Autodesk Inventor part; units mm, degrees
ref_plane "YZ Plane" through (0, 0, 0) normal (1, 0, 0) x (0, 1, 0)
ref_plane "XZ Plane" through (0, 0, 0) normal (0, 1, 0) x (-1, 0, 0)
ref_plane "XY Plane" through (0, 0, 0) normal (0, 0, 1) x (1, 0, 0)
sketch "Sketch1" plane through (0, 0, 0) normal (1, 0, 0) x (0, 1, 0)
  line L0 (-55.5791, 90.9825) -> (55.5791, 90.9825)
  line L1 (55.5791, 90.9825) -> (55.5791, -90.9825)
  line L2 (55.5791, -90.9825) -> (-55.5791, -90.9825)
  line L3 (-55.5791, -90.9825) -> (-55.5791, 90.9825)
  line L4 (-55.5791, 90.9825) -> (55.5791, -90.9825) construction
  line L5 (55.5791, 90.9825) -> (-55.5791, -90.9825) construction
  circle A0 centre (35.8863, -80.1209) radius 6.35
  arc A1 (28.845, 21.2348) -> (-35.1241, -7.4567) centre (35.8863, -80.1209) ccw construction
  arc A2 (28.1849, 30.7369) -> (-41.7813, -0.6445) centre (35.8863, -80.1209) ccw
  arc A3 (29.5052, 11.7327) -> (-28.4669, -14.269) centre (35.8863, -80.1209) ccw
  arc A4 (29.5052, 11.7327) -> (28.1849, 30.7369) centre (28.845, 21.2348) ccw
  arc A5 (-41.7813, -0.6445) -> (-28.4669, -14.269) centre (-35.1241, -7.4567) ccw
  circle A6 centre (28.845, 71.7808) radius 14.2875
  point P0 (0, 0)
  dimension "d2" = 12.7
  dimension "d3" = 101.6
  dimension "d4" = 19.05
  dimension "d5" = 28.575
  dimension "d9" = 50.546
  dimension "d10" = 0
  dimension "d11" = 181.965
  dimension "d12" = 111.1583
extrude "Extrusion1" add sketch "Sketch1" along normal blind 7.9375
properties part number "side_plate" material "Steel"
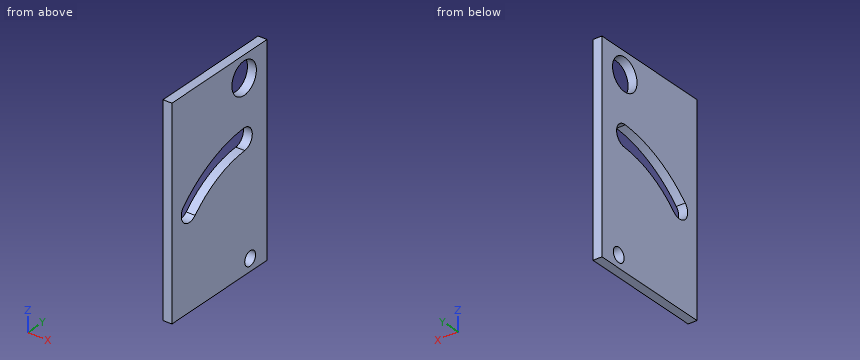
Can you work these out from the model? Positions are in its coordinate system, mm. Round coordinates to 2 decimals unless told otherwise and drop trailing zeros. Write each loop counter-clockwise with the first axis right and the second up, starting at its lowest first coordinate (ties: lowest second). Pieces come first, ordered by that corner, then holes. Notation, with made-up numbers: (-28.5, 24.25) - (-9.5, 24.25) arc R20 ccw to (-9.5, 61.25) - close; hole circle Ø8 at (17, -13). An arc over 180 degrees is marked (long way). Write each question's results on one line, items separated by ' | '. Start each with the question number.
1) Suppose I cut it at D-D (y = 23). List the corners of the cut face in (x, z) for me.
2) Suppose I cut it at B-B (z = -3). List the corners of the cut face in (x, y) for me, and give its area (3 significant figures).
3) Please list where these lines run through material, in increasing order: line 1 (Z direction, x = 2.5, y = 23.5); line 2 (Z direction, x = 2.5, y = 37.5); line 3 (Z direction, x = 7.5, y = 17).
4) Suppose I cut it at A-A (x = 3.25). Give the number of separate pieces and of enclosed holes in the cut face, and give its area (3 significant figures).
5) Suppose I cut it at C-C (y = 36). List the corners of the cut face in (x, z) for me, and give its area (3 significant figures).
Here are the results:
1) outline: (0, -90.98) - (7.94, -90.98) - (7.94, 11.05) - (0, 11.05) - close; (0, 30.25) - (7.94, 30.25) - (7.94, 58.74) - (0, 58.74) - close; (0, 84.82) - (7.94, 84.82) - (7.94, 90.98) - (0, 90.98) - close
2) outline: (0, -55.58) - (7.94, -55.58) - (7.94, -43.54) - (0, -43.54) - close; (0, -14.41) - (7.94, -14.41) - (7.94, 55.58) - (0, 55.58) - close | area: 651 mm2
3) line 1: z = -90.98 to 11.12, 30.31 to 58.53, 85.03 to 90.98 | line 2: z = -90.98 to -86.26, -73.98 to 17.26, 25.21 to 60.41, 83.15 to 90.98 | line 3: z = -90.98 to 10, 29.39 to 63.79, 79.77 to 90.98
4) separate pieces: 1 | enclosed holes: 3 | area: 17,800 mm2
5) outline: (0, -90.98) - (7.94, -90.98) - (7.94, -86.47) - (0, -86.47) - close; (0, -73.77) - (7.94, -73.77) - (7.94, 14.95) - (0, 14.95) - close; (0, 27.52) - (7.94, 27.52) - (7.94, 59.41) - (0, 59.41) - close; (0, 84.15) - (7.94, 84.15) - (7.94, 90.98) - (0, 90.98) - close | area: 1,050 mm2
